Read the model definition and answer for the solid it produces. Units are mm, in the model's axes. A direction names the side the tool comes from. Round coordinates to 2 decimals unless told otherwise and drop trailing zeros. Write each loop counter-clockwise with the first axis right and the second up, starting at its lowest first coordinate (ties: lowest second). Pieces come first, ordered by that corner, then holes. Notation, with made-up numbers: (59, 81.5) -> (79, 81.5) arc R19 cw to (79, 94.5) -> close; hole circle Ø2 at (79, -13.75). An arc over 180 degrees is marked (long way). Return JSON: item names as keys, results as strings. Group by question number.
(1) A cutting plane is placed at C-C on x = 17. Give the vertices of the cut face in (y, z), then the cut area to 3 significant figures.
(2) A cutting plane is placed at D-D on x = 23.5. Give the vertices of the cut face in (y, z), then the cut area to 3 significant figures.
(3) Straight lines are drawn through the part: line 1 (X direction, y = 5, z = 0); line 2 (Z direction, x = 14, y = 7); line 3 (Y direction, x = 9, z = -10). For each, find the intervals that lie inside material, in ascending order.
(4) A cutting plane is placed at B-B on z = 0. Give the vertices of the cut face in (x, y), then the cut area to 4 significant figures.
(5) A cutting plane is placed at A-A on y = 51. Give the vertices of the cut face in (x, z), then the cut area to 3 significant figures.
(6) The mould has two halves that part along Y. Classify faces 4 (the cylindrical face through (18.77, 5.07, -0.62)), 5 (the cylindrical face through (33.03, 38.34, 0.1)), 6 (the flat face through (23, 0, 0)): released by +Y, released by -Y, zero draft, split by the parting line, or undercut.
(7) Given pin 1 (1 mm diameter, centred on y = 56, z = 14.5, fed in from -X); pin 2 (4 mm diameter, centred on x = 17.5, y = 12.5, fed in from +Z); pin 3 (22.5 mm diameter, centred on x = 10, z = -3.5, fed in from +Y), each flat-ended and moving along its own axis, determine where each tip first touches the part or whether it passes through.
(8) For faces 1 (the flat face through (14, 10, 6)), 2 (the flat face through (30, 30, 25.4)), 3 (the flat face through (33, 53, -4.762)), determine the directions among +Z, -Z, +X, -X, +Y, -Y from which every point of the face is accessible in a straight line to the end or side of a thin tool.
```python
from build123d import *

# Parameters (mm, degrees)
EXTRUIR_L_MINA1_DEPTH = 25.4
CROQUIS2_R            = 4.7625
CORTAR_EXTRUIR1_DEPTH = 81.493540113
CORTAR_EXTRUIR2_DEPTH = 10


with BuildPart() as part:
    # Croquis1 → Extruir-Lámina1 (new, symmetric)
    with BuildSketch(Plane.XY):
        Polygon((0, 0), (38.1, 0), (38.1, 76.2), (28.1, 76.2), (28.1, 10), (0, 10), align=None)
    extrude(amount=EXTRUIR_L_MINA1_DEPTH, both=True)

    # Croquis2 → Cortar-Extruir1 (cut, through all)
    with BuildSketch(Plane(origin=(0, 10, 0), x_dir=(1, 0, 0), z_dir=(0, 1, 0))):
        with Locations(Location((14.05, 0, 0), (0, 0, 270))):
            Circle(CROQUIS2_R)
    extrude(amount=-CORTAR_EXTRUIR1_DEPTH, mode=Mode.SUBTRACT)

    # Croquis3 → Cortar-Extruir2 (cut)
    with BuildSketch(Plane.ZY.offset(-28.1)):
        with BuildLine():
            Line((-4.7625, 43.1), (-4.7625, 63.1))
            ThreePointArc((-4.7625, 63.1), (0, 67.8625), (4.7625, 63.1))
            Line((4.7625, 63.1), (4.7625, 43.1))
            ThreePointArc((4.7625, 43.1), (0, 38.3375), (-4.7625, 43.1))
        make_face()
    extrude(amount=-CORTAR_EXTRUIR2_DEPTH, mode=Mode.SUBTRACT)


solid = part.part
```
Checks:
{
 "1": {"outline": "(0, -25.4) -> (10, -25.4) -> (10, -3.74) -> (0, -3.74) -> close; (0, 3.74) -> (10, 3.74) -> (10, 25.4) -> (0, 25.4) -> close", "area": "433 mm^2"},
 "2": {"outline": "(0, -25.4) -> (10, -25.4) -> (10, 25.4) -> (0, 25.4) -> close", "area": "508 mm^2"},
 "3": {"line 1": "x = 0 to 9.29, 18.81 to 38.1", "line 2": "z = -25.4 to -4.76, 4.76 to 25.4", "line 3": "y = 0 to 10"},
 "4": {"outline": "(0, 0) -> (9.29, 0) -> (9.29, 10) -> (0, 10) -> close; (18.81, 0) -> (38.1, 0) -> (38.1, 38.34) -> (28.1, 38.34) -> (28.1, 10) -> (18.81, 10) -> close; (28.1, 67.86) -> (38.1, 67.86) -> (38.1, 76.2) -> (28.1, 76.2) -> close", "area": "652.5 mm^2"},
 "5": {"outline": "(28.1, -25.4) -> (38.1, -25.4) -> (38.1, -4.76) -> (28.1, -4.76) -> close; (28.1, 4.76) -> (38.1, 4.76) -> (38.1, 25.4) -> (28.1, 25.4) -> close", "area": "413 mm^2"},
 "6": {"face 4": "zero draft", "face 5": "undercut", "face 6": "released by -Y"},
 "7": {"pin 1": "stops at x = 28.1", "pin 2": "passes through", "pin 3": "stops at y = 10"},
 "8": {"face 1": "+Z, -Z, -X, +Y", "face 2": "+Z, +X, -X, +Y, -Y", "face 3": "+X, -X"}
}
